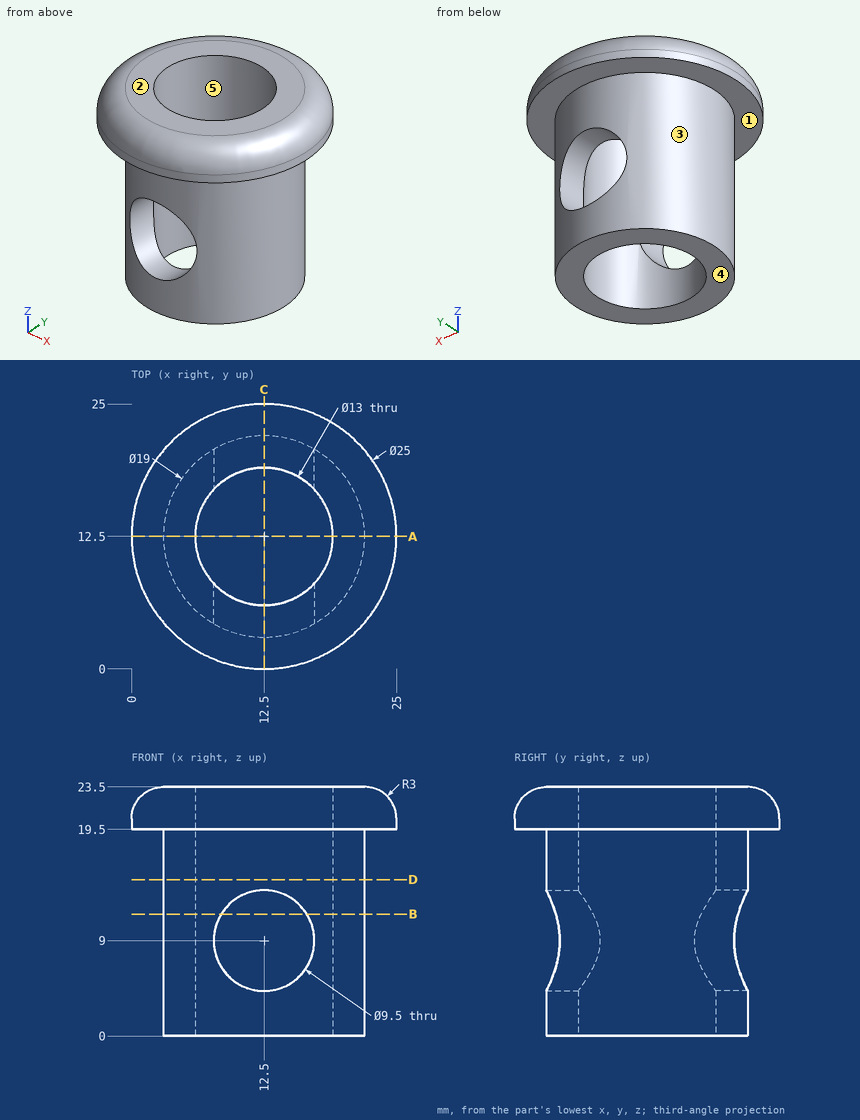
Print and shaded views of the part. All mm, measured from the part's lowest x, y and z. A direction names the side the tool comes from. Coordinates: 2 decimals unless noted, no trailing zeros. Order: outer loops, then holes, each group sorted by start corner. A loop starts at its lowest first (then second) coordinate and runs counter-clockwise, first axis right, second up.
Item 1: Saw through at C-C on x = 12.5. List the corners of the cut face in (y, z).
Filled in:
outline: (0, 19.5) - (3, 19.5) - (3, 13.75) - (6, 13.75) - (6, 23.5) - (3, 23.5) arc R3 ccw to (0, 20.5) - close; (3, 0) - (6, 0) - (6, 4.25) - (3, 4.25) - close; (19, 0) - (22, 0) - (22, 4.25) - (19, 4.25) - close; (19, 13.75) - (22, 13.75) - (22, 19.5) - (25, 19.5) - (25, 20.5) arc R3 ccw to (22, 23.5) - (19, 23.5) - close
Item 2: Saw through at D-D on z = 14.75. List the corners of the cut face in (x, y).
Filled in:
outline: circle Ø19 at (12.5, 12.5); hole circle Ø13 at (12.5, 12.5)
Item 3: Saw through at A-A on y = 12.5. List the corners of the cut face in (x, z), then the cut area to 3 significant figures.
Filled in:
outline: (0, 19.5) - (3, 19.5) - (3, 0) - (6, 0) - (6, 23.5) - (3, 23.5) arc R3 ccw to (0, 20.5) - close; (19, 0) - (22, 0) - (22, 19.5) - (25, 19.5) - (25, 20.5) arc R3 ccw to (22, 23.5) - (19, 23.5) - close
area: 161 mm2
Item 4: Drop flat-ended pins along their axis: pin 1 Ø8 at (x, y) = (12.5, 12.5) entering from -Z; pin 2 Ø4 at (x, z) = (19.5, 10) entering from -Y; pin 3 Ø12 at (x, z) = (9, 4) entering from -Y; pin 4 Ø1.5 at (y, z) = (19, 19) entering from +X. Give the stop position or say it passes through.
Filled in:
pin 1: passes through
pin 2: stops at y = 4.42
pin 3: stops at y = 3
pin 4: stops at x = 23.5
Item 5: Mould opens along X. For the marked faces 3, 4 and 5 say: released by +X, released by -X, zero draft, split by the parting line, or undercut.
Filled in:
face 3: split by the parting line
face 4: zero draft
face 5: undercut
Item 6: Tool access for the marked faces 1 and 2: list every direction of +Z, -Z, +X, -X, +Y, -Y with a clear straight run to the whole face (end or side of a thin tool).
Filled in:
face 1: -Z
face 2: +Z, +X, -X, +Y, -Y
Item 7: Saw through at B-B on z = 11.5. List the corners of the cut face in (x, y), then the cut area to 3 significant figures.
Filled in:
outline: (8.46, 3.9) - (8.46, 7.41) arc R6.5 cw to (8.46, 17.59) - (8.46, 21.1) arc R9.5 ccw to start; (16.54, 3.9) arc R9.5 ccw to (16.54, 21.1) - (16.54, 17.59) arc R6.5 cw to (16.54, 7.41) - close
area: 99.9 mm2
Item 8: Drill centre lines: L1, parallel to Y at x = 12.5, z = 18.5; L2, parallel to Z at x = 12.5, y = 5.75; L3, parallel to Y at x = 9, z = 12.5. Where is each one in solid material? Low to high.
Filled in:
L1: y = 3 to 6, 19 to 22
L2: z = 0 to 4.25, 13.75 to 23.5
L3: y = 3.67 to 7.02, 17.98 to 21.33
